Build history of the part. All positions in model axes, mm. A direction names the side the tool comes from. Coordinates: 2 decimals unless noted, no trailing zeros. Return JSON: item names as keys, results as strings.
from build123d import *

# Parameters (mm, degrees)
SKETCH1_R           = 2
SKETCH1_R_2         = 3.5
SKETCH1_W           = 9
SKETCH1_H           = 2
SKETCH1_W_2         = 5
BOSS_EXTRUDE1_DEPTH = 4


with BuildPart() as part:
    # Sketch1 → Boss-Extrude1 (new body)
    with BuildSketch(Plane.XY):
        with BuildLine():
            Line((-12.978640908, -18), (-12.978640908, -24))
            Line((-12.978640908, -24), (23.021359092, -24))
            Line((23.021359092, -24), (23.021359092, -18))
            ThreePointArc((23.021359092, -18), (32.58126188, -15.140073441), (39, -7.5))
            ThreePointArc((39, -7.5), (45.227131985, 9.097629123), (47.343034567, 26.698237678))
            ThreePointArc((47.343034567, 26.698237678), (46.561018226, 46.955835458), (44.219623828, 67.092858318))
            Line((44.219623828, 67.092858318), (28.140376172, 69.067141682))
            Line((28.140376172, 69.067141682), (26.638766331, 75.523635508))
            Line((26.638766331, 75.523635508), (10.441233669, 75.806364492))
            Line((10.441233669, 75.806364492), (8.1, 82.51))
            Line((8.1, 82.51), (-8.1, 82.51))
            Line((-8.1, 82.51), (-14.491217975, 82.280462515))
            Line((-14.491217975, 82.280462515), (-30.688782025, 81.999537485))
            ThreePointArc((-30.688782025, 81.999537485), (-37.609553588, 47.248902923), (-36.96836533, 11.821617405))
            ThreePointArc((-36.96836533, 11.821617405), (-29.196719191, -6.486518424), (-12.978640908, -18))
        make_face()
        with Locations((38.147341743, 11.821617405)):
            Circle(SKETCH1_R, mode=Mode.SUBTRACT)
        with Locations((-24.678960076, 61.651218734)):
            Circle(SKETCH1_R_2, mode=Mode.SUBTRACT)
        with Locations(Location((1.521420673, 61.651218734, 0), (0, 0, 180))):
            Circle(SKETCH1_R_2, mode=Mode.SUBTRACT)
        with Locations((14.86306514, 46.821617405)):
            Circle(SKETCH1_R_2, mode=Mode.SUBTRACT)
        with Locations(Location((38.147341743, 46.821617405, 0), (0, 0, 180))):
            Circle(SKETCH1_R_2, mode=Mode.SUBTRACT)
        with Locations((-31.681501662, 43.456405989)):
            Circle(SKETCH1_R, mode=Mode.SUBTRACT)
        with Locations((-14, -9.124358763)):
            Circle(SKETCH1_R, mode=Mode.SUBTRACT)
        with Locations((0, 77.51)):
            Rectangle(SKETCH1_W, SKETCH1_H, mode=Mode.SUBTRACT)
        Polygon((-4, -2.5), (0, -2.5), (0, 0), (12, 0), (12, -2.5), (16, -2.5), (16, -12.5), (12, -12.5), (12, -15), (0, -15), (0, -12.5), (-4, -12.5), align=None, mode=Mode.SUBTRACT)
        with Locations((35.147341743, 56.321617405)):
            Rectangle(SKETCH1_W_2, SKETCH1_H, mode=Mode.SUBTRACT)
        Polygon((-27.318093916, 78.057395991), (-18.319447222, 78.213465452), (-18.284765119, 76.213766187), (-27.283411813, 76.057696726), align=None, mode=Mode.SUBTRACT)
        with Locations((17.86306514, 56.399848624)):
            Rectangle(SKETCH1_W_2, SKETCH1_H, mode=Mode.SUBTRACT)
        with Locations((-0.478579327, 71.151218734)):
            Rectangle(SKETCH1_W_2, SKETCH1_H, mode=Mode.SUBTRACT)
        Polygon((14.041615104, 71.742910288), (14.006710291, 69.743214898), (23.005339548, 69.58614324), (23.040244361, 71.58583863), align=None, mode=Mode.SUBTRACT)
        Polygon((40.158980309, 63.561403348), (31.226064944, 64.658227439), (30.982326257, 62.673135135), (39.915241622, 61.576311045), align=None, mode=Mode.SUBTRACT)
        Polygon((1.632632483, 35.912105076), (1.005748572, 29.944943559), (-18.884789816, 32.034556594), (-18.257905905, 38.00171811), align=None, mode=Mode.SUBTRACT)
        with Locations((-22.678960076, 71.151218734)):
            Rectangle(SKETCH1_W_2, SKETCH1_H, mode=Mode.SUBTRACT)
        Polygon((0.065422707, 20.994201285), (-1.188345114, 9.059878252), (-21.078883502, 11.149491286), (-19.825115681, 23.083814319), align=None, mode=Mode.SUBTRACT)
        Polygon((-9.666, 24.072796069), (-9.153, 28.955923243), (-23.205665371, 30.432234852), (-22.787742764, 34.410342529), (-30.743958119, 35.246187743), (-31.161880726, 31.268080066), (-34.143965433, 31.581364852), (-34.656965433, 26.698237678), (-31.674880726, 26.384952891), (-32.092803333, 22.406845214), (-24.136587978, 21.571), (-23.718665371, 25.549107678), align=None, mode=Mode.SUBTRACT)
    extrude(amount=BOSS_EXTRUDE1_DEPTH)


solid = part.part
1. Drop flat-ended pins along their axis: pin 1 (2 mm diameter, centred on y = -20, z = 3, fed in from +X); pin 2 (1.2 mm diameter, centred on y = -14, z = 2, fed in from -X); pin 3 (0.6 mm diameter, centred on y = 71, z = 2, fed in from -X). Give the stop position or say it passes through.
Check values:
{"pin 1": "x = 23.02", "pin 2": "x = -21.84", "pin 3": "x = -33.8"}
2. Cut at A-A on z = 1.65. State how many separate pieces and enclosed holes the cut face has, plus the area to 3 significant figures.
Check values:
{"separate pieces": "1", "enclosed holes": "19", "area": "6,630 mm²"}
3. Tool access for faces 1 (the flat face through (0, 82.51, 2)), 2 (the flat face through (-4, -8, 2)): list every direction of +Z, -Z, +X, -X, +Y, -Y with a clear straight run to the whole face (end or side of a thin tool).
Check values:
{"face 1": "+Z, -Z, +X, -X, +Y", "face 2": "+Z, -Z"}
4. Probe L1, parallel to Y at x = -8, z = 1.85; L2, parallel to Y at x = -25.5, z = 0.35; L3, parallel to Y at x = -30.5, z = 0.2. List the from-to ranges inside material, lowest first.
Check values:
{"L1": "-24 to 9.78, 21.84 to 30.89, 36.92 to 82.51", "L2": "-10.44 to 21.71, 34.7 to 58.25, 65.05 to 76.09, 78.09 to 82.09", "L3": "-4.76 to 22.24, 35.22 to 41.84, 45.07 to 82"}
5. Mould opens along Y. For faces 3 (the flat face through (36.293, 68.066, 1.972)), 4 (the cylindrical face through (32.46, -15.22, 1.97)), 5 (the flat face through (12, -1, 2)) say: pulls with the +Y half, pulls with the -Y half, needs draft (parallel to the pull), parting line crosses it, or undercut.
Check values:
{"face 3": "pulls with the +Y half", "face 4": "pulls with the -Y half", "face 5": "undercut"}
